Geometry: see drawing. Coordinates: mm, zero at the bounding-box minimum. Give positions to 0.01 mm unless a question says otherwise; leave off trailing zeros. Loops run counter-clockwise (first coordinate to the right, second up) from the corner with the lowest first, then second, coordinate; pieces in that order, holes last. Notation, with made-up numbers: M -26,62.5 L 20,62.5 A17 ccw 20,66.5 Z; hole C -34.5,10 d5. An arc over 180 degrees is marked long. Put each result on its own line as item: value.
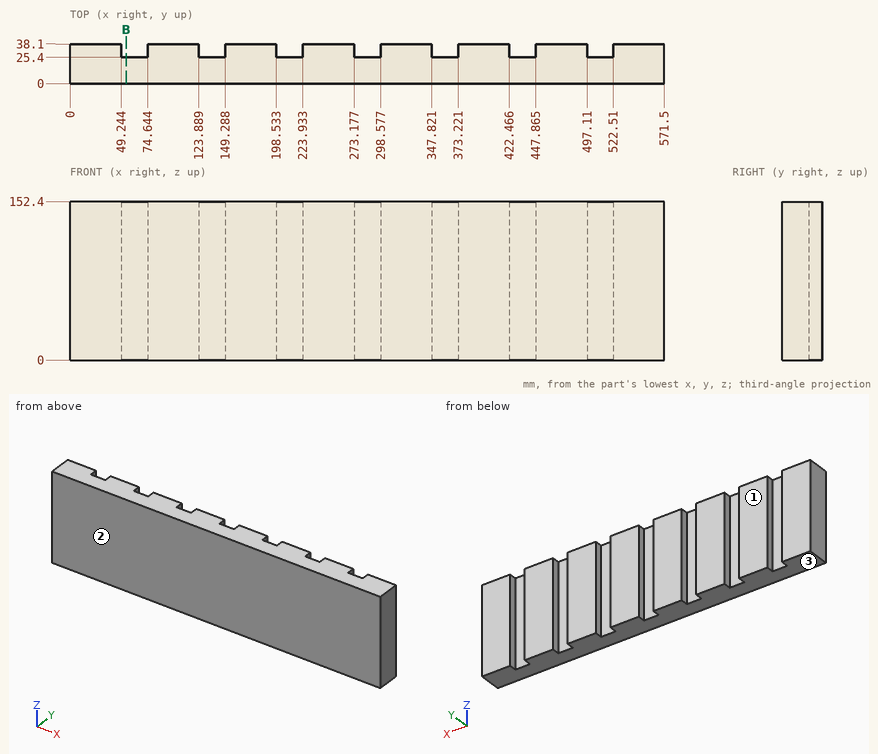
1. Section query B-B (x = 54). Output: boundary loops of the cut face in (y, z).
Found:
outline: M 0,0 L 25.4,0 L 25.4,152.4 L 0,152.4 Z
2. Draft query along Y for the marked faces 1, 2 and 3. Return one class per face: pulls with the +Y half, pulls with the -Y half, needs draft (parallel to the pull), parting line crosses it, or undercut.
Found:
face 1: pulls with the +Y half
face 2: pulls with the -Y half
face 3: needs draft
3. Material intervals for line 1 (Y direction, x = 298, z = 131.5), sorted ascending. Write a range as from..to.
Found:
line 1: 0..25.4
4. Contact query for a flat-ended pin moving along its axis: P1, Ø4, axis at x = 138, z = 40, coming from the +Y side. Output: stop coordinate, or through.
Found:
P1: y = 25.4
